CAD build for the part. Positions are in the model's coordinates, mm. A direction names the side the tool comes from. Coordinates: 2 decimals unless noted, no trailing zeros. Loops run counter-clockwise (first coordinate to the right, second up) from the corner with the lowest first, then second, coordinate; pieces in that order, holes last.
1) Saw through at B-B, the plane x = 35. Write the cut outline in (y, z), and give its area (3 significant figures).
2) Saw through at A-A, the plane z = 35. Write the cut outline in (x, y).
3) Wall check: line 1 along Z through (x, y) = (35, -1.6); line 2 along Y through (x, z) = (-6, -4.5); line 3 along X through (y, z) = (-21, 20). Give the ranges that are in metal, low to high.
4) Saw through at C-C, the plane z = -7. Write the cut outline in (x, y).
5) Which spindle directions (+Z, -Z, +X, -X, +Y, -Y) get a long thin tool onto all of the face, cutting with end or side? Do faces 4 (the flat face through (2, -17, 0)), 5 (the flat face through (-1, 0, 1)), 6 (the flat face through (0, -17, 25)). Say none if no direction does.
6) Two-plate mould, pull along Z, no slides. Class faces 1 (the flat face through (0, -17, -25)), 2 (the cylindrical face through (-33.5, -1.014, 32.117)), 3 (the flat face through (-2, -17, 0)): +Z half, -Z half, draft (parallel to the pull), parting line (faces both ways), or undercut.
7) Saw through at D-D, the plane x = -21. Write the cut outline in (y, z), and give its area (3 significant figures).
8) Pin check, flat tips, straight feed: pin 1 Ø1.2 at (x, y) = (-0.5, -15.5) entering from +Z; pin 2 Ø9 at (y, z) = (-12, -9) entering from +X; pin 3 Ø5 at (x, z) = (-35, -35) entering from -Y (1 decimal); pin 4 Ø4.5 at (x, y) = (-0.5, -11) entering from -Z. Stop position of each tip, or through.
```python
from build123d import *

# Parameters (mm, degrees)
F0_W     = 100
F0_H     = 100
F1_DEPTH = 2
F2_R     = 3.25
F3_DEPTH = 2.001
F4_W     = 4
F4_H     = 50
F5_DEPTH = 30


with BuildPart() as f1:
    # F0 (on Front) → F1 (new body)
    with BuildSketch(Plane.XZ):
        Rectangle(F0_W, F0_H)
    extrude(amount=F1_DEPTH)

    # F2 (on face) → F3 (cut, through all)
    with BuildSketch(Plane.XZ.offset(2)):
        with Locations((-35, 35)):
            Circle(F2_R)
        with Locations((35, 35)):
            Circle(F2_R)
        with Locations((-35, -35)):
            Circle(F2_R)
        with Locations((35, -35)):
            Circle(F2_R)
    extrude(amount=-F3_DEPTH, mode=Mode.SUBTRACT)

    # F4 (on face) → F5 (join)
    with BuildSketch(Plane.XZ.offset(2)):
        Rectangle(F4_W, F4_H)
    extrude(amount=F5_DEPTH)


solid = f1.part
```
Data:
1. outline: (-2, -50) - (0, -50) - (0, -38.25) - (-2, -38.25) - close; (-2, -31.75) - (0, -31.75) - (0, 31.75) - (-2, 31.75) - close; (-2, 38.25) - (0, 38.25) - (0, 50) - (-2, 50) - close
1. area: 174 mm2
2. outline: (-50, -2) - (-38.25, -2) - (-38.25, 0) - (-50, 0) - close; (-31.75, -2) - (31.75, -2) - (31.75, 0) - (-31.75, 0) - close; (38.25, -2) - (50, -2) - (50, 0) - (38.25, 0) - close
3. line 1: z = -50 to -38.25, -31.75 to 31.75, 38.25 to 50
3. line 2: y = -2 to 0
3. line 3: x = -2 to 2
4. outline: (-50, -2) - (-2, -2) - (-2, -32) - (2, -32) - (2, -2) - (50, -2) - (50, 0) - (-50, 0) - close
5. face 4: +Z, -Z, +X, -Y
5. face 5: +Z, -Z, +X, -X, +Y
5. face 6: +Z, +X, -X, -Y
6. face 1: -Z half
6. face 2: undercut
6. face 3: draft
7. outline: (-2, -50) - (0, -50) - (0, 50) - (-2, 50) - close
7. area: 200 mm2
8. pin 1: stops at z = 25
8. pin 2: stops at x = 2
8. pin 3: passes through
8. pin 4: stops at z = -25
